Part model, mm, in its own coordinate system. Give positions to 0.01 mm unless a question says otherwise; leave off trailing zeros. Use one line per item in the form item = value. Start each with the question number.
1. Band-saw the part on A-A, the plane y = -0.9. State how many separate pieces and enclosed holes the cut face has, plus the area to 3 significant figures.
2. Drill centre lines: line 1 (X direction, y = -2.1, z = 90) (3 decimals); line 2 (X direction, y = -0.2, z = 509). Where is each one in solid material? Low to high.
3. Pin check, flat tips, straight feed: P1, Ø3.5, axis at x = 10, z = 370, coming from the +Y side; P2, Ø2.5, axis at x = 10, z = 290, coming from the -Y side. Stop position of each tip, or through.
from build123d import *

# Parameters (mm, degrees)
SKETCH_1_W          = 20
SKETCH_1_H          = 3
EXTRUDE_1_DEPTH     = 640
SKETCH_2_R          = 1.575
CUT_EXTRUDE_1_DEPTH = 641.319451524


with BuildPart() as part:
    # 草图1 → 凸台-拉伸1 (new body)
    with BuildSketch(Plane.XY):
        with Locations((10, -1.5)):
            Rectangle(SKETCH_1_W, SKETCH_1_H)
    extrude(amount=EXTRUDE_1_DEPTH)

    # 草图2 → 切除-拉伸1 (cut, through all)
    with BuildSketch(Plane(origin=(0, 0, 0), x_dir=(1, 0, 0), z_dir=(0, 1, 0))):
        with Locations(Location((10, -10, 0), (0, 0, 270))):
            Circle(SKETCH_2_R)
        with Locations(Location((10, -30, 0), (0, 0, 270))):
            Circle(SKETCH_2_R)
        with Locations(Location((10, -50, 0), (0, 0, 270))):
            Circle(SKETCH_2_R)
        with Locations(Location((10, -70, 0), (0, 0, 270))):
            Circle(SKETCH_2_R)
        with Locations(Location((10, -90, 0), (0, 0, 270))):
            Circle(SKETCH_2_R)
        with Locations(Location((10, -110, 0), (0, 0, 270))):
            Circle(SKETCH_2_R)
        with Locations(Location((10, -130, 0), (0, 0, 270))):
            Circle(SKETCH_2_R)
        with Locations(Location((10, -150, 0), (0, 0, 270))):
            Circle(SKETCH_2_R)
        with Locations(Location((10, -170, 0), (0, 0, 270))):
            Circle(SKETCH_2_R)
        with Locations(Location((10, -190, 0), (0, 0, 270))):
            Circle(SKETCH_2_R)
        with Locations(Location((10, -210, 0), (0, 0, 270))):
            Circle(SKETCH_2_R)
        with Locations(Location((10, -230, 0), (0, 0, 270))):
            Circle(SKETCH_2_R)
        with Locations(Location((10, -250, 0), (0, 0, 270))):
            Circle(SKETCH_2_R)
        with Locations(Location((10, -270, 0), (0, 0, 270))):
            Circle(SKETCH_2_R)
        with Locations(Location((10, -290, 0), (0, 0, 270))):
            Circle(SKETCH_2_R)
        with Locations(Location((10, -310, 0), (0, 0, 270))):
            Circle(SKETCH_2_R)
        with Locations(Location((10, -330, 0), (0, 0, 270))):
            Circle(SKETCH_2_R)
        with Locations(Location((10, -350, 0), (0, 0, 270))):
            Circle(SKETCH_2_R)
        with Locations(Location((10, -370, 0), (0, 0, 270))):
            Circle(SKETCH_2_R)
        with Locations(Location((10, -390, 0), (0, 0, 270))):
            Circle(SKETCH_2_R)
        with Locations(Location((10, -410, 0), (0, 0, 270))):
            Circle(SKETCH_2_R)
        with Locations(Location((10, -430, 0), (0, 0, 270))):
            Circle(SKETCH_2_R)
        with Locations(Location((10, -450, 0), (0, 0, 270))):
            Circle(SKETCH_2_R)
        with Locations(Location((10, -470, 0), (0, 0, 270))):
            Circle(SKETCH_2_R)
        with Locations(Location((10, -490, 0), (0, 0, 270))):
            Circle(SKETCH_2_R)
        with Locations(Location((10, -510, 0), (0, 0, 270))):
            Circle(SKETCH_2_R)
        with Locations(Location((10, -530, 0), (0, 0, 270))):
            Circle(SKETCH_2_R)
        with Locations(Location((10, -550, 0), (0, 0, 270))):
            Circle(SKETCH_2_R)
        with Locations(Location((10, -570, 0), (0, 0, 270))):
            Circle(SKETCH_2_R)
        with Locations(Location((10, -590, 0), (0, 0, 270))):
            Circle(SKETCH_2_R)
        with Locations(Location((10, -610, 0), (0, 0, 270))):
            Circle(SKETCH_2_R)
        with Locations(Location((10, -630, 0), (0, 0, 270))):
            Circle(SKETCH_2_R)
    extrude(amount=-CUT_EXTRUDE_1_DEPTH, mode=Mode.SUBTRACT)


solid = part.part
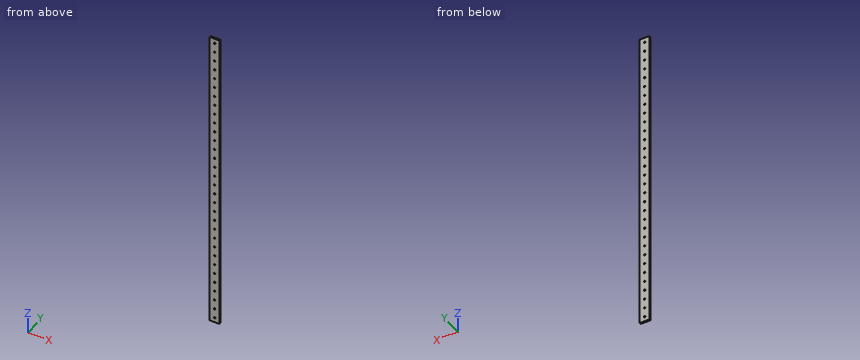
From the geometry:
q1.separate_pieces = 1
q1.enclosed_holes = 32
q1.area = 12,600 mm²
q2.line_1 = 0 to 8.425, 11.575 to 20
q2.line_2 = 0 to 8.78, 11.22 to 20
q3.P1 = 0
q3.P2 = through
